Design review of the part built by this model. Coordinates are the model's own, in mm. Coordinates: 2 decimals unless noted, no trailing zeros. Write each loop counter-clockwise with the first axis right and the second up, starting at its lowest first coordinate (ties: lowest second). Pieces come first, ordered by that corner, then holes. Notation, with made-up numbers: (-39.5, -28) -> (-32.5, -28) arc R21 cw to (-32.5, 11) -> close; hole circle Ø2 at (-31, -12.75). An arc over 180 degrees is marked (long way). Return JSON: item names as keys, results as strings. Group by question number.
from build123d import *

# Parameters (mm, degrees)
ESQUISSE1_W             = 83.5
ESQUISSE1_H             = 90
BOSS_EXTRU_1_DEPTH      = 2
ESQUISSE2_R             = 1
ENL_V_MAT_EXTRU_1_DEPTH = 3
CONG_1_R                = 4
ENL_V_MAT_EXTRU_2_DEPTH = 3


with BuildPart() as part:
    # Esquisse1 → Boss.-Extru.1 (new body)
    with BuildSketch(Plane(origin=(0, 0, 0), x_dir=(1, 0, 0), z_dir=(0, 1, 0))):
        Rectangle(ESQUISSE1_W, ESQUISSE1_H)
    extrude(amount=BOSS_EXTRU_1_DEPTH)

    # Esquisse2 → Enlèv. mat.-Extru.1 (cut, through all)
    with BuildSketch(Plane(origin=(0, 0, 0), x_dir=(1, 0, 0), z_dir=(0, 1, 0))):
        with Locations((-23.75, -25)):
            Circle(ESQUISSE2_R)
        with Locations((-37.75, -25)):
            Circle(ESQUISSE2_R)
        with Locations((-37.75, -41)):
            Circle(ESQUISSE2_R)
        with Locations((-23.75, -41)):
            Circle(ESQUISSE2_R)
        with Locations((-23.75, 41)):
            Circle(ESQUISSE2_R)
        with Locations((-37.75, 41)):
            Circle(ESQUISSE2_R)
        with Locations((-37.75, 25)):
            Circle(ESQUISSE2_R)
        with Locations((-23.75, 25)):
            Circle(ESQUISSE2_R)
        Polygon((41.75, 12), (18.25, 12), (-19.75, 45), (41.75, 45), align=None)
        Polygon((41.75, -12), (18.25, -12), (-19.75, -45), (41.75, -45), align=None)
        Polygon((-41.75, -21), (-19.75, -12), (-19.75, 12), (-41.75, 21), align=None)
        with BuildLine():
            Line((20.75, 9), (23.75, 9))
            ThreePointArc((23.75, 9), (24.75, 8), (23.75, 7))
            Line((23.75, 7), (20.75, 7))
            ThreePointArc((20.75, 7), (19.75, 8), (20.75, 9))
        make_face()
        with BuildLine():
            Line((37.75, 7), (34.75, 7))
            ThreePointArc((34.75, 7), (33.75, 8), (34.75, 9))
            Line((34.75, 9), (37.75, 9))
            ThreePointArc((37.75, 9), (38.75, 8), (37.75, 7))
        make_face()
        with BuildLine():
            Line((20.75, -7), (23.75, -7))
            ThreePointArc((23.75, -7), (24.75, -8), (23.75, -9))
            Line((23.75, -9), (20.75, -9))
            ThreePointArc((20.75, -9), (19.75, -8), (20.75, -7))
        make_face()
        with BuildLine():
            Line((37.75, -9), (34.75, -9))
            ThreePointArc((34.75, -9), (33.75, -8), (34.75, -7))
            Line((34.75, -7), (37.75, -7))
            ThreePointArc((37.75, -7), (38.75, -8), (37.75, -9))
        make_face()
    extrude(amount=ENL_V_MAT_EXTRU_1_DEPTH, mode=Mode.SUBTRACT)

    # Congé1
    cong_1_edges = [part.edges().sort_by_distance(p)[0] for p in [
        (-19.75, 1, -12),
        (-41.75, 1, -45),
        (-41.75, 1, 45),
        (41.75, 1, 12),
        (18.25, 1, 12),
        (-19.75, 1, 45),
        (41.75, 1, -12),
        (-19.75, 1, -45),
        (18.25, 1, -12),
        (-41.75, 1, -21),
        (-41.75, 1, 21),
        (-19.75, 1, 12),
    ]]
    fillet(cong_1_edges, radius=CONG_1_R)

    # Esquisse3 → Enlèv. mat.-Extru.2 (cut, through all)
    with BuildSketch(Plane(origin=(0, 0, 0), x_dir=(1, 0, 0), z_dir=(0, 1, 0))):
        with BuildLine():
            Line((-12.5, 13), (-11.5, 13))
            ThreePointArc((-11.5, 13), (-9.5, 11), (-11.5, 9))
            Line((-11.5, 9), (-12.5, 9))
            ThreePointArc((-12.5, 9), (-14.5, 11), (-12.5, 13))
        make_face()
        with BuildLine():
            Line((10.5, 13), (9.5, 13))
            ThreePointArc((9.5, 13), (7.5, 11), (9.5, 9))
            Line((9.5, 9), (10.5, 9))
            ThreePointArc((10.5, 9), (12.5, 11), (10.5, 13))
        make_face()
        with BuildLine():
            Line((10.5, -13), (9.5, -13))
            ThreePointArc((9.5, -13), (7.5, -11), (9.5, -9))
            Line((9.5, -9), (10.5, -9))
            ThreePointArc((10.5, -9), (12.5, -11), (10.5, -13))
        make_face()
        with BuildLine():
            Line((-12.5, -13), (-11.5, -13))
            ThreePointArc((-11.5, -13), (-9.5, -11), (-11.5, -9))
            Line((-11.5, -9), (-12.5, -9))
            ThreePointArc((-12.5, -9), (-14.5, -11), (-12.5, -13))
        make_face()
    extrude(amount=ENL_V_MAT_EXTRU_2_DEPTH, mode=Mode.SUBTRACT)


solid = part.part
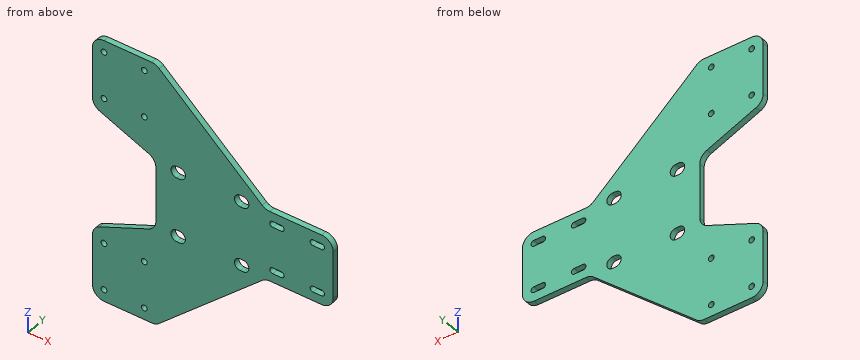
Q1. For P1, Ø3, axis at x = -23.75, z = 41, coming from the +Y side; P2, Ø0.6, axis at x = 28.5, y = 0.5, coming from the +Z side; P3, Ø1.1, axis at x = 10, y = 1.5, coming from the -Z side; P4, Ø0.5, axis at x = 10, y = 1.5, coming from the +Z side, all flat-tipped, find the tip position at first contact; note any pin that passes through.
Q2. We need section D-D on y = 0.3. State how many separate pieces and enclosed holes the cut face has, plus the area to 3 significant figures.
Q3. We need section B-B on x = 27. Write out the cut boundary in (y, z).
Q4. We need section A-A on z = -25. Write out the cut boundary in (x, y), plus the area to 3 significant figures.
Q5. We need section C-C on z = 1. Write out the cut boundary in (x, y).
Q6. Wall thickness on L1, parallel to Z at x = 36.5, y = 1.95; L2, parallel to X at y = 0.6, z = -8; L3, parallel to Z at x = -23.75, y = 0.8: over which ranges is each line inside the solid? List them lowest first.
Findings below:
{
 "1": {"P1": "stops at y = 2", "P2": "stops at z = 12", "P3": "stops at z = -19.64", "P4": "stops at z = 19.38"},
 "2": {"separate pieces": "1", "enclosed holes": "16", "area": "3,840 mm^2"},
 "3": {"outline": "(0, -12) -> (2, -12) -> (2, 12) -> (0, 12) -> close"},
 "4": {"outline": "(-41.75, 0) -> (-38.75, 0) -> (-38.75, 2) -> (-41.75, 2) -> close; (-36.75, 0) -> (-24.75, 0) -> (-24.75, 2) -> (-36.75, 2) -> close; (-22.75, 0) -> (3.28, 0) -> (3.28, 2) -> (-22.75, 2) -> close", "area": "82.1 mm^2"},
 "5": {"outline": "(-19.75, 0) -> (41.75, 0) -> (41.75, 2) -> (-19.75, 2) -> close"},
 "6": {"L1": "z = -12 to -9, -7 to 7, 9 to 12", "L2": "x = -19.75 to 19.75, 24.75 to 33.75, 38.75 to 41.75", "L3": "z = -45 to -42, -40 to -26, -24 to -13.64, 13.64 to 24, 26 to 40, 42 to 45"}
}
